Could you check a few things on this model? Use its own coordinates, in mm. A direction names the side the tool comes from. Give positions to 0.01 mm unless a question says otherwise; leave off trailing zeros. Order: outer loops, then holes, each group sorted by start corner. A loop starts at its lowest first (then second) coordinate and runs counter-clockwise, first axis right, second up.
(1) Will these pins go through, and if not, where does the flat tip stop? pin 1 (2 mm diameter, centred on x = -9, y = -9, fed in from -Z); pin 2 (3 mm diameter, centred on y = -7, z = -4, fed in from -X); pin 3 (0.9 mm diameter, centred on x = -3, y = 4, fed in from -Z); pin 4 (1.6 mm diameter, centred on x = -0.5, z = -10, fed in from +Y).
(2) If I drill on probe 1 along Y at (x, z) = (0, -0.1); probe 2 along Y at (x, z) = (9, -0.45); probe 3 along Y at (x, z) = (-6, 1.5), over which ranges is the centre line in solid material (lowest first)?
(3) Imagine slicing it at C-C, the plane y = -11. Write out the boundary of the cut face in (x, z), then the cut area to 3 significant figures.
(4) If we mould it in two halves opening along X, with no side actions, what happens to faces 4 (the cylindrical face through (-10.016, -9.421, -0.69)), 5 (the cylindrical face through (-12.6, 12.64, -0.69)), 6 (the cylindrical face through (4.82, -2.24, 0.81)), 7 (the flat face through (0, 11, -10))? For each: released by +X, released by -X, zero draft, split by the parting line, or undercut.
(5) Imagine slicing it at A-A, the plane z = 1. State how many separate pieces and enclosed holes the cut face has, then the cut area to 3 significant figures.
(6) On a 3-axis mill with a long thin cutter (end or side, diameter ignored), from which of +Z, -Z, +X, -X, +Y, -Y can I reach the whole of each face in a straight line? I mean faces 1 (the cylindrical face through (-2.6, 4, 0.8)), 2 (the cylindrical face through (0.383, 10.468, -10.724)), 3 (the flat face through (0, 2, -6.4)). Say none if no direction works.
(7) Imagine slicing it at B-B, the plane z = -2.5. Write out the boundary of the cut face in (x, y).
from build123d import *

# Parameters (mm, degrees)
SKETCH_1_R               = 9
EXTRUDE_1_DEPTH          = 2.5
SKETCH_2_R               = 1.1
EXTRUDE_2_DEPTH          = 1.4
SKETCH_3_R               = 10
EXTRUDE_3_DEPTH          = 11.4
SKETCH_4_R               = 8
CUT_EXTRUDE_1_DEPTH      = 4.4
SKETCH_5_R               = 9
CUT_EXTRUDE_2_DEPTH      = 7.4
SKETCH_6_R               = 8
EXTRUDE_4_DEPTH          = 1
SKETCH_7_R               = 0.4
EXTRUDE_5_DEPTH          = 5.5
EXTRUDE_5_DEPTH_BACK     = 10
CHAMFER_1_SIZE           = 0.3
EXTRUDE_START            = 9.949874
SKETCH_8_R               = 1
EXTRUDE_6_DEPTH          = 1.050126
PATTERN_CIRCULAR_1_COUNT = 3


with BuildPart() as part:
    # Эскиз1 → Бобышка-Вытянуть1 (new body)
    with BuildSketch(Plane.XY):
        Circle(SKETCH_1_R)
    extrude(amount=EXTRUDE_1_DEPTH)

    # Эскиз2 → Бобышка-Вытянуть2 (add)
    with BuildSketch(Plane(origin=(0, 0, 0), x_dir=(-1, 0, 0), z_dir=(0, 0, -1))):
        with BuildLine():
            Line((10.5, -13.5), (-10.5, -13.5))
            ThreePointArc((-10.5, -13.5), (-12.621320344, -12.621320344), (-13.5, -10.5))
            Line((-13.5, -10.5), (-13.5, 10.5))
            ThreePointArc((-13.5, 10.5), (-12.621320344, 12.621320344), (-10.5, 13.5))
            Line((-10.5, 13.5), (10.5, 13.5))
            ThreePointArc((10.5, 13.5), (12.621320344, 12.621320344), (13.5, 10.5))
            Line((13.5, 10.5), (13.5, -10.5))
            ThreePointArc((13.5, -10.5), (12.621320344, -12.621320344), (10.5, -13.5))
        make_face()
        with Locations((9, 9)):
            Circle(SKETCH_2_R, mode=Mode.SUBTRACT)
        with Locations((-9, 9)):
            Circle(SKETCH_2_R, mode=Mode.SUBTRACT)
        with Locations((9, -9)):
            Circle(SKETCH_2_R, mode=Mode.SUBTRACT)
        with Locations((-9, -9)):
            Circle(SKETCH_2_R, mode=Mode.SUBTRACT)
    extrude(amount=EXTRUDE_2_DEPTH)

    # Эскиз3 → Бобышка-Вытянуть3 (add)
    with BuildSketch(Plane(origin=(0, 0, -1.4), x_dir=(-1, 0, 0), z_dir=(0, 0, -1))):
        with Locations(Location((0, 0, 0), (0, 0, 180))):
            Circle(SKETCH_3_R)
    extrude(amount=EXTRUDE_3_DEPTH)

    # Эскиз4 → Вырез-Вытянуть1 (cut)
    with BuildSketch(Plane.XY.offset(2.5)):
        Circle(SKETCH_4_R)
    extrude(amount=-CUT_EXTRUDE_1_DEPTH, mode=Mode.SUBTRACT)

    # Эскиз5 → Вырез-Вытянуть2 (cut)
    with BuildSketch(Plane(origin=(0, 0, -12.8), x_dir=(-1, 0, 0), z_dir=(0, 0, -1))):
        with Locations(Location((0, 0, 0), (0, 0, 180))):
            Circle(SKETCH_5_R)
    extrude(amount=-CUT_EXTRUDE_2_DEPTH, mode=Mode.SUBTRACT)

    # Эскиз6 → Бобышка-Вытянуть4 (add)
    with BuildSketch(Plane(origin=(0, 0, -5.4), x_dir=(-1, 0, 0), z_dir=(0, 0, -1))):
        with Locations(Location((0, 0, 0), (0, 0, 180))):
            Circle(SKETCH_6_R)
    extrude(amount=EXTRUDE_4_DEPTH)

    # Эскиз7 → Бобышка-Вытянуть5 (add, two sides)
    with BuildSketch(Plane(origin=(0, 0, -6.4), x_dir=(-1, 0, 0), z_dir=(0, 0, -1))) as extrude_5_sk:
        Circle(SKETCH_7_R)
        with Locations((3, 0)):
            Circle(SKETCH_7_R)
        with Locations((6, 0)):
            Circle(SKETCH_7_R)
        with Locations((4.5, 2)):
            Circle(SKETCH_7_R)
        with Locations((-3, 0)):
            Circle(SKETCH_7_R)
        with Locations((-6, 0)):
            Circle(SKETCH_7_R)
        with Locations((-4.5, 2)):
            Circle(SKETCH_7_R)
        with Locations((-1.5, 2)):
            Circle(SKETCH_7_R)
        with Locations((1.5, 2)):
            Circle(SKETCH_7_R)
        with Locations((-3, 4)):
            Circle(SKETCH_7_R)
        with Locations((3, 4)):
            Circle(SKETCH_7_R)
        with Locations((0, 4)):
            Circle(SKETCH_7_R)
        with Locations((0, -4)):
            Circle(SKETCH_7_R)
        with Locations((3, -4)):
            Circle(SKETCH_7_R)
        with Locations((-3, -4)):
            Circle(SKETCH_7_R)
        with Locations((1.5, -2)):
            Circle(SKETCH_7_R)
        with Locations((-1.5, -2)):
            Circle(SKETCH_7_R)
        with Locations((-4.5, -2)):
            Circle(SKETCH_7_R)
        with Locations((4.5, -2)):
            Circle(SKETCH_7_R)
    extrude(amount=EXTRUDE_5_DEPTH)
    extrude(extrude_5_sk.sketch, amount=-EXTRUDE_5_DEPTH_BACK)

    # Фаска1
    chamfer_1_edges = [part.edges().sort_by_distance(p)[0] for p in [
        (-10, 0, -12.8),
        (-8, 0, 2.5),
        (-9, 0, 2.5),
        (-9, 0, -12.8),
    ]]
    chamfer(chamfer_1_edges, length=CHAMFER_1_SIZE)

    # Эскиз8 → Бобышка-Вытянуть6 (add)
    with BuildSketch(Plane(origin=(0, 0, 0), x_dir=(1, 0, 0), z_dir=(0, 1, 0)).offset(EXTRUDE_START)):
        with Locations(Location((0, 9.8, 0), (0, 0, 90))):
            Circle(SKETCH_8_R)
    extrude_6 = extrude(amount=EXTRUDE_6_DEPTH)

    # Круговой массив1: Бобышка-Вытянуть6 ×3 about axis
    pattern_circular_1_axis = Axis((0, 0, 0), (0, 0, 1))
    for i in range(1, PATTERN_CIRCULAR_1_COUNT):
        add(extrude_6.rotate(pattern_circular_1_axis, i * 360 / PATTERN_CIRCULAR_1_COUNT))


solid = part.part
Answer block:
1. pin 1: passes through
1. pin 2: stops at x = -8.35
1. pin 3: stops at z = -11.9
1. pin 4: stops at y = 11
2. probe 1: y = -13.5 to -8, -4.4 to -3.6, -0.4 to 0.4, 3.6 to 4.4, 8 to 13.5
2. probe 2: y = -13.5 to -10.1, -7.9 to 7.9, 10.1 to 13.5
2. probe 3: y = -6.71 to -5.29, -0.4 to 0.4, 5.29 to 6.71
3. outline: (-13.46, -1.4) - (13.46, -1.4) - (13.46, 0) - (-13.46, 0) - close
3. area: 37.7 mm2
4. face 4: undercut
4. face 5: released by -X
4. face 6: undercut
4. face 7: zero draft
5. separate pieces: 20
5. enclosed holes: 1
5. area: 63.0 mm2
6. face 1: +Z
6. face 2: +Y
6. face 3: -Z
7. outline: circle Ø20 at (0, 0)
